Read the model definition and answer for the solid it produces. Units are mm, in the model's axes. A direction names the side the tool comes from. Coordinates: 2 decimals unless noted, no trailing zeros. Order: outer loops, then holes, each group sorted by start corner. A loop starts at its lowest first (then second) coordinate and runs counter-clockwise, first axis right, second up. Notation, with made-up numbers: (71, 48.25) - (117, 48.25) arc R24 ccw to (117, 80.25) - close; hole circle Ø1 at (30, 68.25). An arc over 180 degrees is marked (long way). Write item = value, one per line.
from build123d import *

# Parameters (mm, degrees)
F0_R     = 29.464
F0_R_2   = 5.715
F0_R_3   = 1.651
F1_DEPTH = 7.62
F0_R_4   = 33.274
F2_DEPTH = 11.811


# Not quite as in the source:
# - a fillet or chamfer that OpenCascade refuses, or shapes differently, is made with other operations: its cross-section is extruded or revolved along the edge and cut away or added


with BuildPart() as f1:
    # F0 (on Front) → F1 (new body, symmetric)
    with BuildSketch(Plane.XZ):
        Circle(F0_R)
        with Locations((-13.2907790592, -13.2907790592)):
            Circle(F0_R_2, mode=Mode.SUBTRACT)
        with Locations((0, -18.796)):
            Circle(F0_R_2, mode=Mode.SUBTRACT)
        with Locations((13.2907790592, -13.2907790592)):
            Circle(F0_R_2, mode=Mode.SUBTRACT)
        with Locations((-18.796, 0)):
            Circle(F0_R_2, mode=Mode.SUBTRACT)
        with Locations((-13.2907790592, 13.2907790592)):
            Circle(F0_R_2, mode=Mode.SUBTRACT)
        Circle(F0_R_3, mode=Mode.SUBTRACT)
        with Locations((13.2907790592, 13.2907790592)):
            Circle(F0_R_2, mode=Mode.SUBTRACT)
        with Locations((18.796, 0)):
            Circle(F0_R_2, mode=Mode.SUBTRACT)
        with Locations((0, 18.796)):
            Circle(F0_R_2, mode=Mode.SUBTRACT)
    extrude(amount=F1_DEPTH, both=True)

    # F0 (on Front) → F2 (join, symmetric)
    with BuildSketch(Plane.XZ):
        Circle(F0_R_4)
        Circle(F0_R, mode=Mode.SUBTRACT)
    extrude(amount=F2_DEPTH, both=True)

    # F3: fillet of radius 5.08 on 3 edges, made by hand

    # F3_s1 → F3_t2 (revolve, cut)
    with BuildSketch(Plane.XY):
        with BuildLine():
            ThreePointArc((33.274, 6.8923111503), (32.2100926284, 10.0031631237), (29.464, 11.811))
            Line((29.464, 11.811), (33.274, 11.811))
            Line((33.274, 11.811), (33.274, 6.8923111503))
        make_face()
    revolve(axis=Axis((0, 11.811, 0), (0, -1, 0)), mode=Mode.SUBTRACT)

    # F3_s3 → F3_t4 (revolve, cut)
    with BuildSketch(Plane.XY):
        with BuildLine():
            ThreePointArc((33.274, -6.8923111503), (32.2100926284, -10.0031631237), (29.464, -11.811))
            Line((29.464, -11.811), (33.274, -11.811))
            Line((33.274, -11.811), (33.274, -6.8923111503))
        make_face()
    revolve(axis=Axis((0, -11.811, 0), (0, -1, 0)), mode=Mode.SUBTRACT)


solid = f1.part
1) Determine the mould class of faces 1 (the face through (-4.33, -0.1, 32.99)), 2 (the face through (13.596, -9.686, -26.14)) for opening direction X: pulls with the +X half, pulls with the -X half, needs draft (parallel to the pull), parting line crosses it, or undercut.
Returned:
face_1 = parting line crosses it
face_2 = undercut
2) The part is cut by section A-A (x = 0). Determine the outline of the cut face in (y, z), and give its area (3 significant figures).
Returned:
outline = (-11.81, -29.46) arc R5.08 ccw to (-6.89, -33.27) - (6.89, -33.27) arc R5.08 ccw to (11.81, -29.46) - (7.62, -29.46) - (7.62, -24.51) - (-7.62, -24.51) - (-7.62, -29.46) - close; (-11.81, 29.46) - (-7.62, 29.46) - (-7.62, 24.51) - (7.62, 24.51) - (7.62, 29.46) - (11.81, 29.46) arc R5.08 ccw to (6.89, 33.27) - (-6.89, 33.27) arc R5.08 ccw to start; (-7.62, -13.08) - (7.62, -13.08) - (7.62, -1.65) - (-7.62, -1.65) - close; (-7.62, 1.65) - (7.62, 1.65) - (7.62, 13.08) - (-7.62, 13.08) - close
area = 660 mm^2
3) The part is cut by section B-B (z = 0). Determine the outline of the cut face in (x, y), and give its area (3 significant figures).
Returned:
outline = (-33.27, -6.89) arc R5.08 ccw to (-29.46, -11.81) - (-29.46, -7.62) - (-24.51, -7.62) - (-24.51, 7.62) - (-29.46, 7.62) - (-29.46, 11.81) arc R5.08 ccw to (-33.27, 6.89) - close; (-13.08, -7.62) - (-1.65, -7.62) - (-1.65, 7.62) - (-13.08, 7.62) - close; (1.65, -7.62) - (13.08, -7.62) - (13.08, 7.62) - (1.65, 7.62) - close; (24.51, -7.62) - (29.46, -7.62) - (29.46, -11.81) arc R5.08 ccw to (33.27, -6.89) - (33.27, 6.89) arc R5.08 ccw to (29.46, 11.81) - (29.46, 7.62) - (24.51, 7.62) - close
area = 660 mm^2
4) Straight lines are drawn through the part: line 1 along Z through (x, y) = (14.5, 2.5); line 2 along X through (y, z) = (3.75, -11.5); line 3 along Y through (x, z) = (-22, 11.5). For each, find the intervals that lie inside material, in ascending order. Write a range as from..to.
Returned:
line_1 = -29.95..-18.88, -7.71..-3.77, 3.77..7.71, 18.88..29.95
line_2 = -31.22..-18.72, -7.86..7.86, 18.72..31.22
line_3 = -7.62..7.62
5) Flat-ended cylindrical pins translate along their axes: pin 1 Ø2 at (y, z) = (-0.5, 24.5) entering from +X; pin 2 Ø2 at (x, z) = (25, -11.5) entering from +Y; pin 3 Ø18.5 at (x, z) = (13.29, 13.29) entering from -Y. Find the tip coordinate at first contact, or state that the pin passes through.
Returned:
pin_1 = 23.56
pin_2 = 7.62
pin_3 = -7.62
6) For faces 3 (the face through (13.596, 9.745, -26.14)), 4 (the face through (6, -7.62, 0)), 5 (the face through (18.74, 0.11, 15.01)), determine the directions among +Z, -Z, +X, -X, +Y, -Y from which every point of the face is accessible in a straight line to the end or side of a thin tool.
Returned:
face_3 = +Y
face_4 = -Y
face_5 = +Y, -Y
